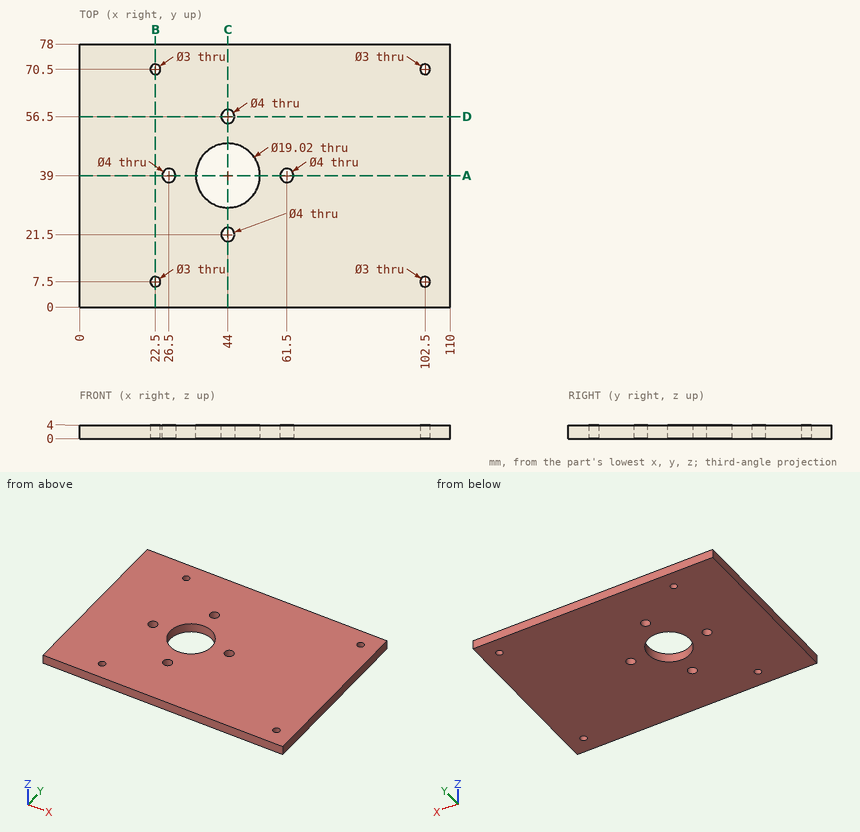
Check sheet for the drawn part. Datum: minimum x, y, z corner. Units: mm. Round coordinates to 2 decimals unless told otherwise and drop trailing zeros. Order: outer loops, then holes, each group sorted by start corner. A loop starts at its lowest first (then second) coordinate and runs counter-clockwise, first axis right, second up.
1) Section check D-D (y = 56.5). Record the boundary of the cut face in (x, z).
2) Scan lines: line 1 (Y direction, x = 22.5, z = 3.1); line 2 (Y direction, x = 44, z = 2.2); line 3 (Y direction, x = 61.5, z = 3.1). Record each from-to range of solid material in increasing order.
3) Section check A-A (y = 39). Record the boundary of the cut face in (x, z).
4) Go/stop test with a flat-tipped pin: pin 1 Ø2.5 at (x, y) = (26.5, 39) entering from +Z. Record where the tip stops, or that it passes through.
5) Section check B-B (x = 22.5). Record the boundary of the cut face in (y, z), and give its area (3 significant figures).
6) Section check C-C (x = 44). Record the boundary of the cut face in (y, z), and give its area (3 significant figures).
Result:
1. outline: (0, 0) - (42, 0) - (42, 4) - (0, 4) - close; (46, 0) - (110, 0) - (110, 4) - (46, 4) - close
2. line 1: y = 0 to 6, 9 to 69, 72 to 78
2. line 2: y = 0 to 19.5, 23.5 to 29.49, 48.51 to 54.5, 58.5 to 78
2. line 3: y = 0 to 37, 41 to 78
3. outline: (0, 0) - (24.5, 0) - (24.5, 4) - (0, 4) - close; (28.5, 0) - (34.49, 0) - (34.49, 4) - (28.5, 4) - close; (53.51, 0) - (59.5, 0) - (59.5, 4) - (53.51, 4) - close; (63.5, 0) - (110, 0) - (110, 4) - (63.5, 4) - close
4. pin 1: passes through
5. outline: (0, 0) - (6, 0) - (6, 4) - (0, 4) - close; (9, 0) - (69, 0) - (69, 4) - (9, 4) - close; (72, 0) - (78, 0) - (78, 4) - (72, 4) - close
5. area: 288 mm2
6. outline: (0, 0) - (19.5, 0) - (19.5, 4) - (0, 4) - close; (23.5, 0) - (29.49, 0) - (29.49, 4) - (23.5, 4) - close; (48.51, 0) - (54.5, 0) - (54.5, 4) - (48.51, 4) - close; (58.5, 0) - (78, 0) - (78, 4) - (58.5, 4) - close
6. area: 204 mm2
